CAD build for the part. Positions are in the model's coordinates, mm. A direction names the side the tool comes from. Give positions to 0.01 mm unless a question says otherwise; leave off trailing zeros. Loops run counter-clockwise (first coordinate to the right, second up) from the corner with the lowest first, then second, coordinate; pieces in that order, holes last. Notation, with made-up numbers: (46.5, 51) -> (73.5, 51) arc R23 ccw to (73.5, 69) -> close; hole circle Ø9 at (80, 43.25). An arc over 180 degrees is marked (long way). Use one line per item in the form item = value.
```python
from build123d import *

# Parameters (mm, degrees)
F1_DEPTH = 70
F2_ANGLE = 90


with BuildPart() as f1:
    # F0 (on Top) → F1 (new body)
    with BuildSketch(Plane.XY):
        with BuildLine():
            Line((43, 0), (7, 0))
            ThreePointArc((7, 0), (2.0502525317, -2.0502525317), (0, -7))
            Line((0, -7), (0, -43))
            ThreePointArc((0, -43), (2.0502525317, -47.9497474683), (7, -50))
            Line((7, -50), (43, -50))
            ThreePointArc((43, -50), (47.9497474683, -47.9497474683), (50, -43))
            Line((50, -43), (50, -7))
            ThreePointArc((50, -7), (47.9497474683, -2.0502525317), (43, 0))
        make_face()
        with BuildLine():
            ThreePointArc((1, -8), (3.0502525317, -3.0502525317), (8, -1))
            Line((8, -1), (42, -1))
            ThreePointArc((42, -1), (46.9497474683, -3.0502525317), (49, -8))
            Line((49, -8), (49, -42))
            ThreePointArc((49, -42), (46.9497474683, -46.9497474683), (42, -49))
            Line((42, -49), (8, -49))
            ThreePointArc((8, -49), (3.0502525317, -46.9497474683), (1, -42))
            Line((1, -42), (1, -8))
        make_face(mode=Mode.SUBTRACT)
    extrude(amount=-F1_DEPTH)


with BuildPart() as f1_1:
    # F2: moved
    add(f1.part.rotate(Axis((25, 0, 0), (1, 0, 0)), F2_ANGLE))


solid = f1_1.part
```
1. Drill centre lines: line 1 (Z direction, x = 23, y = 46); line 2 (X direction, y = 47, z = -17.5); line 3 (X direction, y = 51, z = -5). Where is each one in solid material? Low to high.
Result sheet:
line_1 = -50 to -49, -1 to 0
line_2 = 0 to 1, 49 to 50
line_3 = 0.29 to 1.68, 48.32 to 49.71
2. Cut at C-C, the plane y = 7. Write the cut outline in (x, z), then the cut area to 3 significant figures.
Result sheet:
outline = (0, -43) arc R7 ccw to (7, -50) -> (43, -50) arc R7 ccw to (50, -43) -> (50, -7) arc R7 ccw to (43, 0) -> (7, 0) arc R7 ccw to (0, -7) -> close; hole (1, -42) arc R7 ccw to (8, -49) -> (42, -49) arc R7 ccw to (49, -42) -> (49, -8) arc R7 ccw to (42, -1) -> (8, -1) arc R7 ccw to (1, -8) -> close
area = 196 mm^2
3. Cut at B-B, the plane z = -30.5. Write the cut outline in (x, y).
Result sheet:
outline = (0, 0) -> (1, 0) -> (1, 70) -> (0, 70) -> close; (49, 0) -> (50, 0) -> (50, 70) -> (49, 70) -> close
4. Tool access for faces 4 (the cylindrical face through (2.1, 34.5, -2)), 5 (the flat face through (25, 35, -1)): list every direction of +Z, -Z, +X, -X, +Y, -Y with a clear straight run to the whole face (end or side of a thin tool).
Result sheet:
face_4 = +Z, -X, +Y, -Y
face_5 = +Y, -Y
5. Cut at A-A, the plane x = 16. Write the cut outline in (y, z).
Result sheet:
outline = (0, -50) -> (70, -50) -> (70, -49) -> (0, -49) -> close; (0, -1) -> (70, -1) -> (70, 0) -> (0, 0) -> close
6. Mould opens along Z. For faces 1 (the cylindrical face through (48, 34.5, -2.1)), 2 (the flat face through (50, 35, -25)), 3 (the cylindrical face through (46.9, 34.5, -3)) say: pulls with the +Z half, pulls with the -Z half, needs draft (parallel to the pull), parting line crosses it, or undercut.
Result sheet:
face_1 = pulls with the +Z half
face_2 = needs draft
face_3 = undercut
